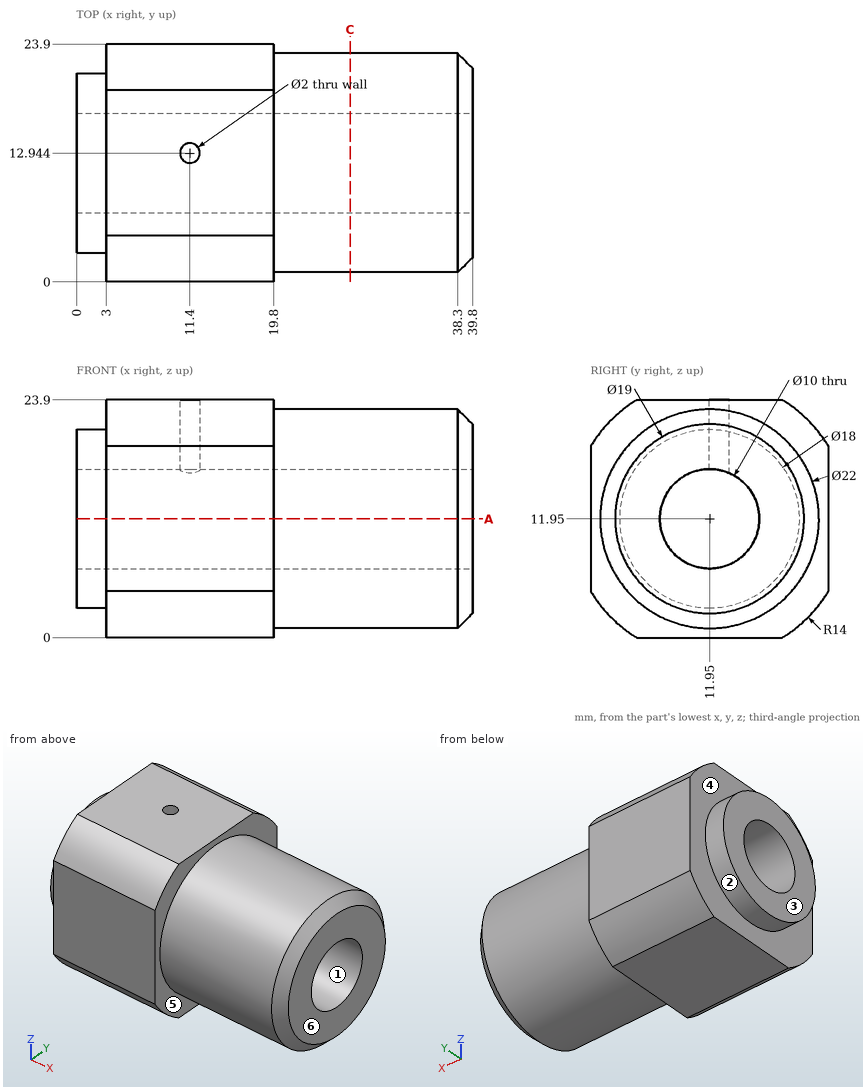
Geometry: see drawing. Coordinates: mm, zero at the bounding-box minimum. A direction names the side the tool comes from. Coordinates: 2 decimals unless noted, no trailing zeros. Loops run counter-clockwise (first coordinate to the right, second up) from the corner with the lowest first, then second, coordinate; pieces in that order, holes last. Notation, with made-up numbers: M 87.25,24.25 L 141.25,24.25 A11 cw 141.25,40.25 Z; hole C -18,-14 d11. An arc over 180 degrees is marked long. Answer in a Markdown table with one row per item.
1. Section A-A, the plane z = 11.95. Output: boundary loops of the cut face in (x, y), then the cut area to 3 significant figures.
Response:
| item | result |
|---|---|
| outline | M 0,2.95 L 3,2.95 L 3,0 L 19.8,0 L 19.8,0.95 L 38.3,0.95 L 39.8,2.45 L 39.8,6.95 L 0,6.95 Z; M 0,16.95 L 39.8,16.95 L 39.8,21.45 L 38.3,22.95 L 19.8,22.95 L 19.8,23.9 L 3,23.9 L 3,20.95 L 0,20.95 Z |
| area | 495 mm2 |
2. Material intervals for line 1 (Y direction, x = 19.5, z = 11.95); line 2 (Y direction, x = 11.4, z = 19); line 3 (Z direction, x = 19.5, y = 9.25), sorted ascending.
Response:
| item | result |
|---|---|
| line 1 | y = 0 to 6.95, 16.95 to 23.9 |
| line 2 | y = 0 to 11.94, 13.94 to 23.9 |
| line 3 | z = 0 to 7.74, 16.16 to 23.9 |
3. Reachability of the marked faces 4, 5 and 6 from +Z, -Z, +X, -X, +Y, -Y: full face, straight path, thin tool, end or side. Return the list, or none.
Response:
| item | result |
|---|---|
| face 4 | -X |
| face 5 | +X |
| face 6 | +Z, -Z, +X, +Y, -Y |
4. Section C-C, the plane x = 27.5. Output: boundary loops of the cut face in (y, z), then the cut area to 3 significant figures.
Response:
| item | result |
|---|---|
| outline | C 11.95,11.95 d22; hole C 11.95,11.95 d10 |
| area | 302 mm2 |
5. First-contact query: pin 1 (1.5 mm diameter, centred on x = 14.5, z = 20.5, fed in from +Y) (1 decimal); pin 2 (8 mm diameter, centred on x = 28.5, y = 7.5, fed in from -Z); pin 3 (1.5 mm diameter, centred on x = 32, z = 13, fed in from -Y). Flat tips, straight axial feed; report the tip coordinate or a pass-through.
Response:
| item | result |
|---|---|
| pin 1 | stops at y = 23.6 |
| pin 2 | stops at z = 0.96 |
| pin 3 | stops at y = 0.95 |
6. Draft query along Y for the marked faces 1, 2 and 3. Return one class per face: pulls with the +Y half, pulls with the -Y half, needs draft (parallel to the pull), parting line crosses it, or undercut.
Response:
| item | result |
|---|---|
| face 1 | undercut |
| face 2 | parting line crosses it |
| face 3 | needs draft |
